Verification items for the finished model (mm, model axes). Face numbers are marked on the shaded views. Round coordinates to 2 decimals unless told otherwise and drop trailing zeros. Write each loop counter-clockwise with the first axis right and the second up, starting at its lowest first coordinate (ties: lowest second). Pieces come first, ordered by that corner, then holes. Notation, with made-up numbers: (34, 0.5) - (49, 0.5) arc R17 ccw to (49, 19.5) - close; hole circle Ø4 at (49, -30.5). An arc over 180 degrees is marked (long way). Write each question's results on one line, items separated by ' | '.
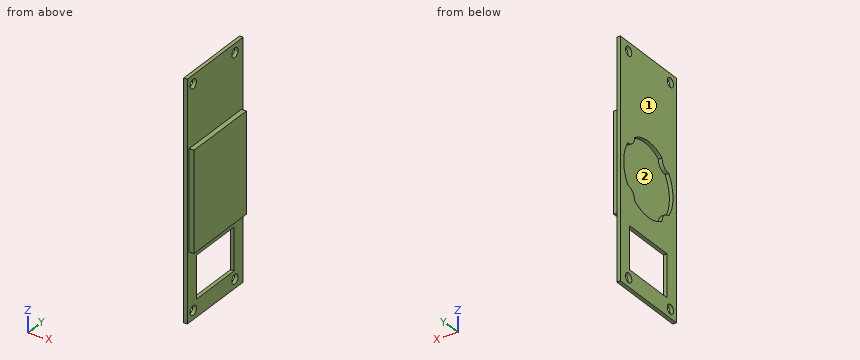
```python
from build123d import *

# Parameters (mm, degrees)
SKETCH1_W           = 122.428
SKETCH1_H           = 43.18
BOSS_EXTRUDE1_DEPTH = 1.905
SKETCH2_R           = 2.413
CUT_EXTRUDE1_DEPTH  = 1.905
CUT_EXTRUDE2_DEPTH  = 1.905
SKETCH4_W           = 21.971
SKETCH4_H           = 28.956
CUT_EXTRUDE3_DEPTH  = 1.905
SKETCH5_W           = 51.6678832
SKETCH5_H           = 40.386705486
BOSS_EXTRUDE2_DEPTH = 2.54


with BuildPart() as part:
    # Sketch1 → Boss-Extrude1 (new body)
    with BuildSketch(Plane(origin=(0, 0, 0), x_dir=(0, 0, -1), z_dir=(1, 0, 0))):
        Rectangle(SKETCH1_W, SKETCH1_H)
    extrude(amount=-BOSS_EXTRUDE1_DEPTH)

    # Sketch2 → Cut-Extrude1 (cut)
    with BuildSketch(Plane(origin=(0, 0, 0), x_dir=(0, 0, -1), z_dir=(1, 0, 0))):
        with Locations((-56.642, 15.24)):
            Circle(SKETCH2_R)
        with Locations((-56.642, -17.018)):
            Circle(SKETCH2_R)
        with Locations((56.642, 15.24)):
            Circle(SKETCH2_R)
        with Locations((56.642, -17.018)):
            Circle(SKETCH2_R)
    extrude(amount=-CUT_EXTRUDE1_DEPTH, mode=Mode.SUBTRACT)

    # Sketch3 → Cut-Extrude2 (cut)
    with BuildSketch(Plane(origin=(0, 0, 0), x_dir=(0, 0, -1), z_dir=(1, 0, 0))):
        with BuildLine():
            ThreePointArc((-10.636223834, -15.804215974), (0, -19.05), (10.636223834, -15.804215974))
            ThreePointArc((10.636223834, -15.804215974), (12.123345763, -12.123345763), (15.804215974, -10.636223834))
            ThreePointArc((15.804215974, -10.636223834), (19.05, 0), (15.804215974, 10.636223834))
            ThreePointArc((15.804215974, 10.636223834), (12.123345763, 12.123345763), (10.636223834, 15.804215974))
            ThreePointArc((10.636223834, 15.804215974), (0, 19.05), (-10.636223834, 15.804215974))
            ThreePointArc((-10.636223834, 15.804215974), (-12.123345763, 12.123345763), (-15.804215974, 10.636223834))
            ThreePointArc((-15.804215974, 10.636223834), (-19.05, 0), (-15.804215974, -10.636223834))
            ThreePointArc((-15.804215974, -10.636223834), (-12.123345763, -12.123345763), (-10.636223834, -15.804215974))
        make_face()
    extrude(amount=-CUT_EXTRUDE2_DEPTH, mode=Mode.SUBTRACT)

    # Sketch4 → Cut-Extrude3 (cut)
    with BuildSketch(Plane.ZY.offset(1.905)):
        with Locations((-41.2115, 0)):
            Rectangle(SKETCH4_W, SKETCH4_H)
    extrude(amount=-CUT_EXTRUDE3_DEPTH, mode=Mode.SUBTRACT)

    # Sketch5 → Boss-Extrude2 (add)
    with BuildSketch(Plane(origin=(0, 0, 0), x_dir=(0, 0, -1), z_dir=(1, 0, 0))):
        Rectangle(SKETCH5_W, SKETCH5_H)
    extrude(amount=BOSS_EXTRUDE2_DEPTH)


solid = part.part
```
(1) Section check A-A (z = -35.5). Record the cut outline in (x, y) (3 decimals), plus the area to 3 significant figures.
Answer:
outline: (-1.905, -21.59) - (0, -21.59) - (0, -14.478) - (-1.905, -14.478) - close; (-1.905, 14.478) - (0, 14.478) - (0, 21.59) - (-1.905, 21.59) - close | area: 27.1 mm2
(2) Go/stop test with flat-tipped pins: pin 1 Ø1.3 at (x, y) = (1.5, -2) entering from +Z; pin 2 Ø2 at (y, z) = (16.5, 46) entering from +X; pin 3 Ø0.8 at (x, z) = (1, -10.5) entering from +Y. Record where each tip stops, or that it passes through.
Answer:
pin 1: z = 25.83 | pin 2: x = 0 | pin 3: y = 20.19
(3) Section check B-B (y = -9.5). Record the cut outline in (x, z) (3 decimals).
Answer:
outline: (-1.905, -61.214) - (0, -61.214) - (0, -52.197) - (-1.905, -52.197) - close; (-1.905, -30.226) - (0, -30.226) - (0, -25.834) - (2.54, -25.834) - (2.54, 25.834) - (0, 25.834) - (0, 61.214) - (-1.905, 61.214) - (-1.905, 16.512) - (0, 16.512) - (0, -16.512) - (-1.905, -16.512) - close
(4) Section check D-D (x = 1). Record the cut outline in (y, z), plus the area to 3 significant figures.
Answer:
outline: (-20.19, -25.83) - (20.19, -25.83) - (20.19, 25.83) - (-20.19, 25.83) - close | area: 2,090 mm2
(5) Mould release check, pull along Y, two halves, no side actions. Record for the marked faces 1 and 2: released by +Y, released by -Y, zero draft, split by the parting line, or undercut.
Answer:
face 1: zero draft | face 2: undercut
(6) Thickness scan on L1, parallel to Z at x = -1, y = 14; L2, parallel to Y at x = -1, z = -37.5; L3, parallel to Z at x = 2.15, y = -15. Record the ranges inside material, lowest first.
Answer:
L1: -61.21 to -58.71, -54.57 to -52.2, -30.23 to -10.93, 10.93 to 54.57, 58.71 to 61.21 | L2: -21.59 to -14.48, 14.48 to 21.59 | L3: -25.83 to 25.83
(7) Section check C-C (z = 18). Record the cut outline in (x, y) (3 decimals), plus the area to 3 significant figures.
Answer:
outline: (-1.905, -21.59) - (0, -21.59) - (0, -20.193) - (2.54, -20.193) - (2.54, 20.193) - (0, 20.193) - (0, 21.59) - (-1.905, 21.59) - (-1.905, 6.237) - (0, 6.237) - (0, -6.237) - (-1.905, -6.237) - close | area: 161 mm2
